Part print with two shaded views. Sizes in mm from the minimum x, y, z corner. A direction names the side the tool comes from. Round coordinates to 2 decimals unless told otherwise and drop trailing zeros. Order: outer loops, then holes, each group sorted by start corner. A loop starts at its lowest first (then second) coordinate and runs counter-clockwise, first axis right, second up. Notation, with made-up numbers: M 89,-23.5 L 111,-23.5 A18 ccw 111,-3.5 Z; hole C 72.5,1 d10. An arc over 180 degrees is marked long. Put each result on its own line as item: value.
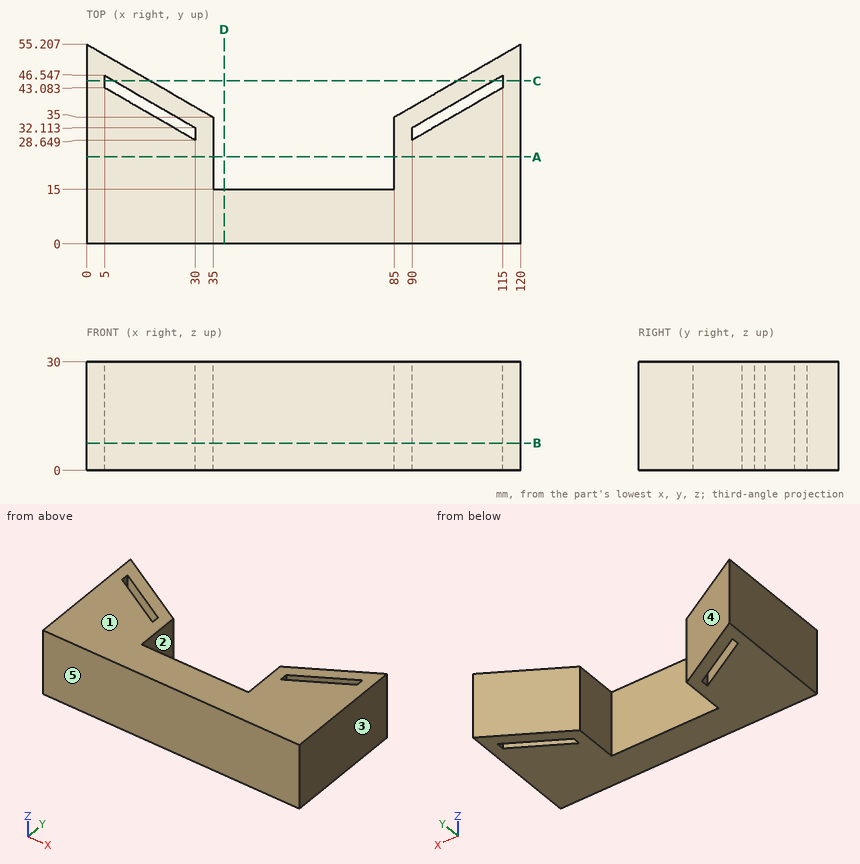
Item 1: Tool access for the marked faces 1 and 2: list every direction of +Z, -Z, +X, -X, +Y, -Y with a clear straight run to the whole face (end or side of a thin tool).
Answers below:
face 1: +Z, +X, -X, +Y, -Y
face 2: +Z, -Z, +Y
Item 2: Band-saw the part on B-B on z = 7.5. Give the cut face in (x, y), and give its area (3 significant figures).
Answers below:
outline: M 0,0 L 120,0 L 120,55.21 L 85,35 L 85,15 L 35,15 L 35,35 L 0,55.21 Z; hole M 5,43.08 L 30,28.65 L 30,32.11 L 5,46.55 Z; hole M 90,28.65 L 115,43.08 L 115,46.55 L 90,32.11 Z
area: 3,730 mm²
Item 3: Band-saw the part on C-C on y = 45. Give the cut face in (x, z), and give its area (3 significant figures).
Answers below:
outline: M 0,0 L 5,0 L 5,30 L 0,30 Z; M 7.68,0 L 17.68,0 L 17.68,30 L 7.68,30 Z; M 102.32,0 L 112.32,0 L 112.32,30 L 102.32,30 Z; M 115,0 L 120,0 L 120,30 L 115,30 Z
area: 900 mm²
Item 4: Pin check, flat tips, straight feed: P1, Ø4, axis at y = 44.5, z = 13.5, coming from the -X side; P2, Ø8, axis at x = 30.5, y = 45, coming from the -Z side; P3, Ø15, axis at x = 48.5, z = 19.5, coming from the +Y side. Stop position of each tip, or through.
Answers below:
P1: x = 0
P2: through
P3: y = 15
Item 5: Band-saw the part on D-D on x = 38. Give the cut face in (y, z), and give its area (3 significant figures).
Answers below:
outline: M 0,0 L 15,0 L 15,30 L 0,30 Z
area: 450 mm²
Item 6: Probe line 1 along X through (y, z) = (24, 17.5); line 2 along X through (y, z) = (44.5, 15.75) (1 decimal); line 3 along X through (y, z) = (40, 13.5). List the from-to ranges inside material, lowest first. Write a range as [from, to].
Answers below:
line 1: [0, 35], [85, 120]
line 2: [0, 5], [8.5, 18.5], [101.5, 111.5], [115, 120]
line 3: [0, 10.34], [16.34, 26.34], [93.66, 103.66], [109.66, 120]
Item 7: Mould opens along X. For the marked faces 3, 4 and 5 say: pulls with the +X half, pulls with the -X half, needs draft (parallel to the pull), parting line crosses it, or undercut.
Answers below:
face 3: pulls with the +X half
face 4: undercut
face 5: needs draft
Item 8: Band-saw the part on A-A on y = 24. Give the cut face in (x, z), and give its area (3 significant figures).
Answers below:
outline: M 0,0 L 35,0 L 35,30 L 0,30 Z; M 85,0 L 120,0 L 120,30 L 85,30 Z
area: 2,100 mm²
